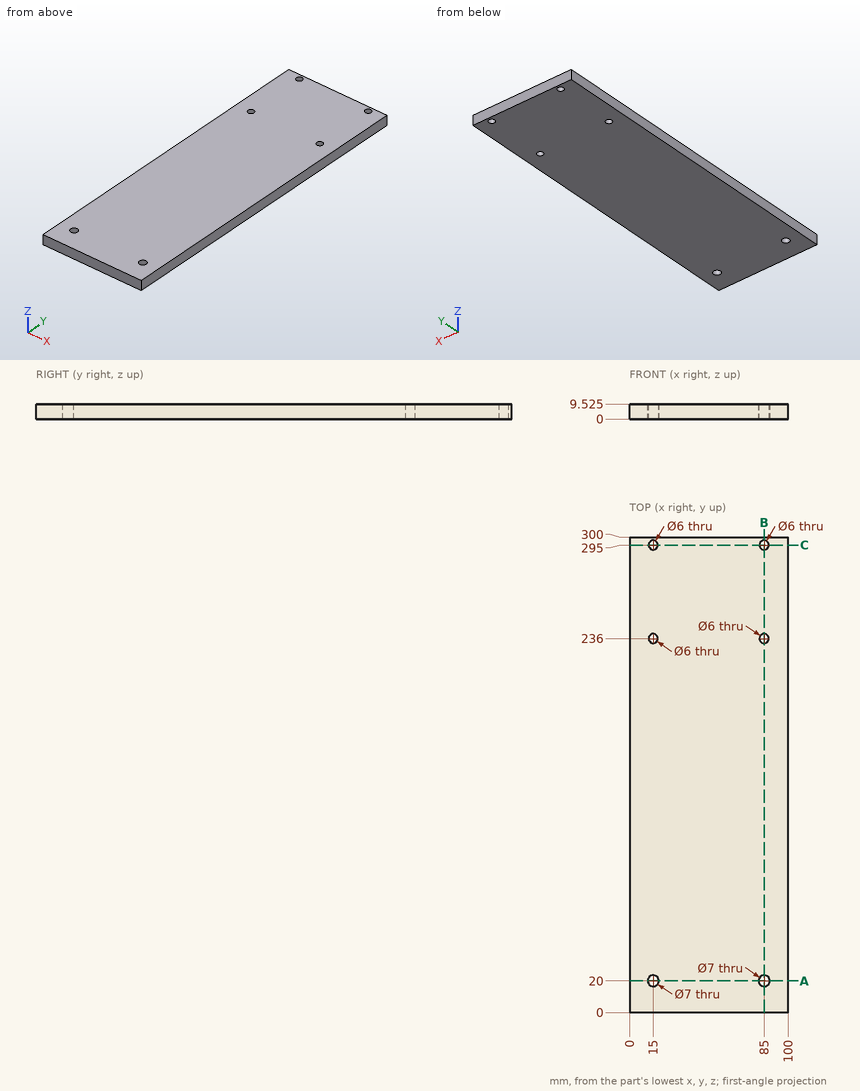
For this review, use the dimensioned drawing (mm, ordinates from the lowest corner) and the shaded views. Round coordinates to 2 decimals unless told otherwise and drop trailing zeros. Order: outer loops, then holes, each group sorted by start corner. A loop starts at its lowest first (then second) coordinate and runs counter-clockwise, first axis right, second up.
1) Consider section A-A (y = 20). State the section outline as (x, z) points (3 decimals).
The answers:
outline: (0, 0) - (11.5, 0) - (11.5, 9.525) - (0, 9.525) - close; (18.5, 0) - (81.5, 0) - (81.5, 9.525) - (18.5, 9.525) - close; (88.5, 0) - (100, 0) - (100, 9.525) - (88.5, 9.525) - close
2) Consider section B-B (x = 85). State the section outline as (y, z) points (3 decimals), plus the area to 3 significant figures.
The answers:
outline: (0, 0) - (16.5, 0) - (16.5, 9.525) - (0, 9.525) - close; (23.5, 0) - (233, 0) - (233, 9.525) - (23.5, 9.525) - close; (239, 0) - (292, 0) - (292, 9.525) - (239, 9.525) - close; (298, 0) - (300, 0) - (300, 9.525) - (298, 9.525) - close
area: 2,680 mm2
3) Consider section C-C (y = 295). State the section outline as (x, z) points (3 decimals), plus the area to 3 significant figures.
The answers:
outline: (0, 0) - (12, 0) - (12, 9.525) - (0, 9.525) - close; (18, 0) - (82, 0) - (82, 9.525) - (18, 9.525) - close; (88, 0) - (100, 0) - (100, 9.525) - (88, 9.525) - close
area: 838 mm2
4) Clearance check with a flat-ended pin moving along its axis: pin 1 Ø3.5 at (x, y) = (15, 295) entering from +Z. State where the tip first meets the part, or that it passes through.
The answers:
pin 1: passes through
5) For L1, parallel to X at y = 295, z = 3; L2, parallel to Y at x = 85, z = 6.75; L3, parallel to X at y = 20, z = 6.25, list the stretches that pass through material, from the lowest coordinate up.
The answers:
L1: x = 0 to 12, 18 to 82, 88 to 100
L2: y = 0 to 16.5, 23.5 to 233, 239 to 292, 298 to 300
L3: x = 0 to 11.5, 18.5 to 81.5, 88.5 to 100
